Here's how the part is built. I have some questions about the finished solid (model axes, mm). Face numbers are marked on the shaded views. A direction names the side the tool comes from. Round coordinates to 2 decimals unless told otherwise and drop trailing zeros. Write each loop counter-clockwise with the first axis right and the second up, starting at its lowest first coordinate (ties: lowest second). Pieces come first, ordered by that corner, then holes. Notation, with made-up numbers: (6, 16.5) -> (17, 16.5) arc R13 cw to (17, 29.5) -> close; hole circle Ø4 at (52, 71). An arc over 180 degrees is marked (long way). Put each result on its own line as item: value. Start each with the question number.
1) If I drill on line 1 along Z through (x, y) = (0, 2.75); line 2 along Y through (x, z) = (10.5, 8); line 3 along X through (y, z) = (1.4, 0), over which ranges is the centre line in solid material (lowest first)? Write a range as [from, to].
2) Will these pins go through, and if not, where does the flat tip stop? P1, Ø10.5, axis at x = 1, z = 34.5, coming from the +Y side; P2, Ø4, axis at x = -0.5, z = 26, coming from the +Y side; P3, Ø12, axis at x = 4.5, z = 22.5, coming from the +Y side.
3) I want a section at A-A, the plane z = 24.5. List the corners of the cut face in (x, y) for me, then the cut area to 3 significant figures.
4) Which directions (+Z, -Z, +X, -X, +Y, -Y) give clear straight access to the entire face, cutting with the end or side of a thin tool? Please do the marked faces 1, 2, 3, 4 and 5.
5) I want a section at B-B, the plane y = 1.25. List the corners of the cut face in (x, z) for me.
from build123d import *
from build123d.topology import SkipClean

# Parameters (mm, degrees)
BOSS_EXTRUDE1_DEPTH = 8
SKETCH2_W           = 9.571982136
SKETCH2_H           = 10
BOSS_EXTRUDE2_DEPTH = 2
BOSS_EXTRUDE3_DEPTH = 9.571982
FILLET1_R           = 2
FILLET2_R           = 4
FILLET3_R           = 2
SKETCH4_W           = 9.571982136
SKETCH4_H           = 1.647948381
BOSS_EXTRUDE4_DEPTH = 6


with BuildPart() as part:
    # Sketch1 → Boss-Extrude1 (new body)
    with BuildSketch(Plane(origin=(0, 0, 0), x_dir=(1, 0, 0), z_dir=(0, 1, 0))):
        with BuildLine():
            Line((-4.785991068, -8.780335386), (-4.785991068, -20.052065634))
            Line((-4.785991068, -20.052065634), (4.785991068, -20.052065634))
            Line((4.785991068, -20.052065634), (4.785991068, -14.215987109))
            ThreePointArc((4.785991068, -14.215987109), (10.931257236, 10.271689989), (-13.891030007, 5.660325552))
            ThreePointArc((-13.891030007, 5.660325552), (-12.461541016, 2.832721051), (-9.365408089, 3.505585733))
            ThreePointArc((-9.365408089, 3.505585733), (9.370244872, 3.492636688), (-4.785991068, -8.780335386))
        make_face()
    extrude(amount=BOSS_EXTRUDE1_DEPTH)

    # Sketch2 → Boss-Extrude2 (add)
    with BuildSketch(Plane.XZ):
        with Locations((0, 25.052065634)):
            Rectangle(SKETCH2_W, SKETCH2_H)
    extrude(amount=-BOSS_EXTRUDE2_DEPTH)

    # Sketch3 → Boss-Extrude3 (add)
    with SkipClean():  # the faces are left unmerged after this step: merging them gives an invalid solid
        with BuildSketch(Plane.ZY.offset(4.785991068)):
            Polygon((28.052065634, 2), (30.052065634, 2), (30.052065634, 5.352051619), (34.052065634, 5.352051619), (34.052065634, 7), (28.052065634, 7), align=None)
        extrude(amount=-BOSS_EXTRUDE3_DEPTH)

    # Fillet1
    fillet1_edges = [part.edges().sort_by_distance(p)[0] for p in [
        (-6.8e-08, 7, 28.052065634),
    ]]
    fillet(fillet1_edges, radius=FILLET1_R)

    # Fillet2
    fillet2_edges = [part.edges().sort_by_distance(p)[0] for p in [
        (0, 8, 20.052065634),
    ]]
    fillet(fillet2_edges, radius=FILLET2_R)

    # Fillet3
    fillet3_edges = [part.edges().sort_by_distance(p)[0] for p in [
        (9.370244872, 8, -3.492636688),
        (10.931257236, 8, -10.271689989),
    ]]
    fillet(fillet3_edges, radius=FILLET3_R)

    # Sketch4 → Boss-Extrude4 (add)
    with BuildSketch(Plane.XY.offset(34.052065634)):
        with Locations((0, 6.17602581)):
            Rectangle(SKETCH4_W, SKETCH4_H)
    extrude(amount=BOSS_EXTRUDE4_DEPTH)


solid = part.part
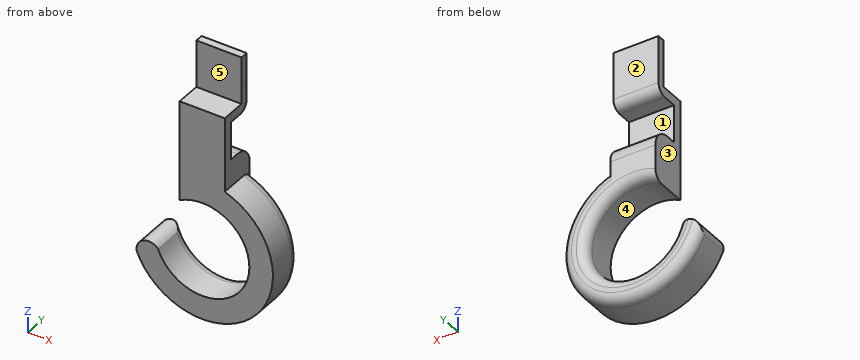
Findings:
1. line 1: z = [-15, -10], [10, 20.05], [28.05, 30.05]
1. line 2: y = [0, 7.99]
1. line 3: x = [10, 15]
2. P1: stops at y = 7
2. P2: stops at y = 2
2. P3: stops at y = 7.97
3. outline: (-4.79, 0) -> (4.79, 0) -> (4.79, 2) -> (-4.79, 2) -> close
3. area: 19.1 mm2
4. face 1: +X, -X, +Y
4. face 2: +Z, +X, -X, +Y
4. face 3: +Z, -X, +Y, -Y
4. face 4: +Y, -Y
4. face 5: +Z, +X, -X, -Y
5. outline: (-13.89, -5.66) arc R15 ccw (long way) to (4.79, 14.22) -> (4.79, 30.05) -> (-4.79, 30.05) -> (-4.79, 8.78) arc R10 cw (long way) to (-9.37, -3.51) arc R2.59 ccw to start
